Geometry check sheet. Reference: the model listing, model coordinates, mm. A direction names the side the tool comes from. Round coordinates to 2 decimals unless told otherwise and drop trailing zeros. Loops run counter-clockwise (first coordinate to the right, second up) from the corner with the lowest first, then second, coordinate; pieces in that order, holes last.
```python
from build123d import *

# Parameters (mm, degrees)
F0_W          = 22
F0_H          = 12
F1_DEPTH      = 22
F2_R          = 2.5
F3_DEPTH      = 4
F4_W          = 12
F4_H          = 3
F5_DEPTH      = 5
F5_DEPTH_BACK = 27
F8_D          = 2.5


with BuildPart() as f1:
    # F0 (on Top) → F1 (new body)
    with BuildSketch(Plane.XY):
        Rectangle(F0_W, F0_H)
    extrude(amount=F1_DEPTH)

    # F2 (on face) → F3 (join)
    with BuildSketch(Plane.XY.offset(22)):
        with BuildLine():
            ThreePointArc((0.428571, -2.555506), (5, 0), (0.428571, 2.555506))
            ThreePointArc((0.428571, 2.555506), (-11, 0), (0.428571, -2.555506))
        make_face()
        with Locations((-5, 0)):
            Circle(F2_R, mode=Mode.SUBTRACT)
    extrude(amount=F3_DEPTH)

    # F4 (on face) → F5 (join, two sides)
    with BuildSketch(Plane(origin=(-11, 0, 0), x_dir=(0, -1, 0), z_dir=(-1, 0, 0))) as f5_sk:
        with Locations((0, 16.5)):
            Rectangle(F4_W, F4_H)
    extrude(amount=F5_DEPTH)
    extrude(f5_sk.sketch, amount=-F5_DEPTH_BACK)

    # F8 (through all)
    with Locations(Plane.XY.offset(18)):
        with Locations((13.5, 0), (-13.5, 0)):
            Hole(F8_D / 2)


solid = f1.part
```
1) Gauge pin test, flat ends, axial feed: pin 1 (2.5 mm diameter, centred on x = -14, y = 2, fed in from -Z); pin 2 (4 mm diameter, centred on x = 14.5, y = -2, fed in from +Z); pin 3 (4.5 mm diameter, centred on y = -0.5, z = 20.5, fed in from -X). Record the tip position at first contact, or that the pin passes through.
Report:
pin 1: stops at z = 15
pin 2: stops at z = 18
pin 3: stops at x = -11
2) Sectioned sample at D-D, the plane z = 11.25. Record the cut outline in (x, y).
Report:
outline: (-11, -6) - (11, -6) - (11, 6) - (-11, 6) - close
3) Sectioned sample at B-B, the plane x = 2. Record the cut outline in (y, z), then the cut area to 3 significant figures.
Report:
outline: (-6, 0) - (6, 0) - (6, 22) - (3, 22) - (3, 26) - (-3, 26) - (-3, 22) - (-6, 22) - close
area: 288 mm2
4) Sectioned sample at A-A, the plane x = -13.5. Record the cut outline in (y, z).
Report:
outline: (-6, 15) - (-1.25, 15) - (-1.25, 18) - (-6, 18) - close; (1.25, 15) - (6, 15) - (6, 18) - (1.25, 18) - close
5) Access from +Z, -Z, +X, -X, +Y, -Y to the whole of each face (thin tool, end or side, straight path). Record for faces 1 (the face through (-13.46, 1.42, 18)), 2 (the face through (11, 0, 20)), 3 (the face through (-11, 0, 7)), 4 (the face through (-2.615, 0.751, 23.972)), 5 (the face through (-10, 5, 22)).
Report:
face 1: +Z, -X, +Y, -Y
face 2: +Z, +X, +Y, -Y
face 3: -Z, -X, +Y, -Y
face 4: +Z
face 5: +Z, -X, +Y
6) Scan lines: line 1 along Z through (x, y) = (7, -5); line 2 along Y through (x, z) = (13.5, 15.85); line 3 along X through (y, z) = (3, 6.25). Record each from-to range of solid material in increasing order.
Report:
line 1: z = 0 to 22
line 2: y = -6 to -1.25, 1.25 to 6
line 3: x = -11 to 11
7) Sectioned sample at C-C, the plane y = 4. Record the cut outline in (x, z).
Report:
outline: (-16, 15) - (-11, 15) - (-11, 0) - (11, 0) - (11, 15) - (16, 15) - (16, 18) - (11, 18) - (11, 22) - (-0.53, 22) - (-0.53, 26) - (-9.47, 26) - (-9.47, 22) - (-11, 22) - (-11, 18) - (-16, 18) - close
